Here's how the part is built. I have some questions about the finished solid (model axes, mm). A direction names the side the tool comes from. Round coordinates to 2 decimals unless told otherwise and drop trailing zeros. Write each loop counter-clockwise with the first axis right and the second up, starting at its lowest first coordinate (ties: lowest second). Pieces come first, ordered by that corner, then holes. Notation, with made-up numbers: (19, 40) -> (43, 40) arc R26 cw to (43, 56) -> close; hole circle Ø1 at (25.25, -21). An arc over 180 degrees is marked (long way). Answer as CSV lines item,"result".
from build123d import *

# Parameters (mm, degrees)
SKETCH_1_R          = 19
SKETCH_1_R_2        = 17.5
EXTRUDE_1_DEPTH     = 80
SKETCH_3_R          = 19
SKETCH_2_R          = 17
SKETCH_4_R          = 17
CUT_EXTRUDE_1_DEPTH = 5


with BuildPart() as part:
    # Эскиз1 → Бобышка-Вытянуть1 (new body)
    with BuildSketch(Plane(origin=(0, 0, 0), x_dir=(1, 0, 0), z_dir=(0, 1, 0))):
        Circle(SKETCH_1_R)
        Circle(SKETCH_1_R_2, mode=Mode.SUBTRACT)
    extrude(amount=EXTRUDE_1_DEPTH)

    # Эскиз3 → По сечениям1 section 0
    with BuildSketch(Plane(origin=(0, 80, 0), x_dir=(1, 0, 0), z_dir=(0, 1, 0))):
        Circle(SKETCH_3_R)
    # Эскиз2 → По сечениям1 section 1
    with BuildSketch(Plane(origin=(0, 85, 0), x_dir=(1, 0, 0), z_dir=(0, 1, 0))):
        Circle(SKETCH_2_R)
    loft()

    # Эскиз4 → Вырез-Вытянуть1 (cut)
    with BuildSketch(Plane(origin=(0, 85, 0), x_dir=(1, 0, 0), z_dir=(0, 1, 0))):
        Circle(SKETCH_4_R)
    extrude(amount=-CUT_EXTRUDE_1_DEPTH, mode=Mode.SUBTRACT)


solid = part.part
Item 1: Suppose I cut it at B-B, the plane y = 73. List the corners of the cut face in (x, z) for me, then the cut area to 3 significant figures.
Results found:
outline,"circle Ø38 at (0, 0); hole circle Ø35 at (0, 0)"
area,"172 mm²"
Item 2: Will these pins go through, and if not, where does the flat tip stop? pin 1 (5 mm diameter, centred on x = 11.5, y = 11, fed in from +Z); pin 2 (6 mm diameter, centred on y = 10.5, z = -7.5, fed in from +X); pin 3 (1 mm diameter, centred on x = -13, z = 10, fed in from +Y); pin 4 (6 mm diameter, centred on y = 40, z = -8, fed in from -X).
Results found:
pin 1,"stops at z = 16.73"
pin 2,"stops at x = 18.46"
pin 3,"passes through"
pin 4,"stops at x = -18.33"
Item 3: If we mould it in two halves opening along X, with no side actions, what happens to faces 1 (the cylindrical face through (-13.887, 39.44, 10.648)), 2 (the flat face through (6, 0, 17)), 3 (the cylindrical face through (8.767, 39.44, 16.856))? For each: pulls with the +X half, pulls with the -X half, needs draft (parallel to the pull), parting line crosses it, or undercut.
Results found:
face 1,"undercut"
face 2,"needs draft"
face 3,"parting line crosses it"
Item 4: Suppose I cut it at A-A, the plane x = 0. List the corners of the cut face in (y, z) for me.
Results found:
outline,"(0, -19) -> (80, -19) -> (85, -17) -> (80, -17) -> (80, -17.5) -> (0, -17.5) -> close; (0, 17.5) -> (80, 17.5) -> (80, 17) -> (85, 17) -> (80, 19) -> (0, 19) -> close"
Item 5: I need wall thicknesses on L1, parallel to X at y = 62, z = 0; L2, parallel to Z at x = 0.5, y = 78; L3, parallel to X at y = 24, z = 4.5. Which ranges of each line are inside material? Lowest first, please.
Results found:
L1,"x = -19 to -17.5, 17.5 to 19"
L2,"z = -18.99 to -17.49, 17.49 to 18.99"
L3,"x = -18.46 to -16.91, 16.91 to 18.46"
Item 6: For faces 4 (the cylindrical face through (9.139, 82.535, -14.334)), 5 (the flat face through (-3, 80, -17)), which set-ups out of +Z, -Z, +X, -X, +Y, -Y let a thin tool reach every point of the face, with its end or its side?
Results found:
face 4,"+Y, -Y"
face 5,"-Y"
